```python
from build123d import *

# Parameters (mm, degrees)
F0_R     = 6
F1_DEPTH = 90


with BuildPart() as f1:
    # F0 (on Top) → F1 (new body)
    with BuildSketch(Plane.XY):
        with BuildLine():
            Line((17.5, 125), (17.5, 112.5))
            ThreePointArc((17.5, 112.5), (0, 95), (-17.5, 112.5))
            Line((-17.5, 112.5), (-17.5, 125))
            ThreePointArc((-17.5, 125), (-63.109528, 109.308909), (-99.503175, 77.655445))
            Line((-99.503175, 77.655445), (-88.677858, 71.405445))
            ThreePointArc((-88.677858, 71.405445), (-82.272413, 47.5), (-106.177858, 41.094555))
            Line((-106.177858, 41.094555), (-117.003175, 47.344555))
            ThreePointArc((-117.003175, 47.344555), (-126.219056, 0), (-117.003175, -47.344555))
            Line((-117.003175, -47.344555), (-106.177858, -41.094555))
            ThreePointArc((-106.177858, -41.094555), (-82.272413, -47.5), (-88.677858, -71.405445))
            Line((-88.677858, -71.405445), (-99.503175, -77.655445))
            ThreePointArc((-99.503175, -77.655445), (-63.109528, -109.308909), (-17.5, -125))
            Line((-17.5, -125), (-17.5, -112.5))
            ThreePointArc((-17.5, -112.5), (0, -95), (17.5, -112.5))
            Line((17.5, -112.5), (17.5, -125))
            ThreePointArc((17.5, -125), (63.109528, -109.308909), (99.503175, -77.655445))
            Line((99.503175, -77.655445), (88.677858, -71.405445))
            ThreePointArc((88.677858, -71.405445), (82.272413, -47.5), (106.177858, -41.094555))
            Line((106.177858, -41.094555), (117.003175, -47.344555))
            ThreePointArc((117.003175, -47.344555), (126.219056, 0), (117.003175, 47.344555))
            Line((117.003175, 47.344555), (106.177858, 41.094555))
            ThreePointArc((106.177858, 41.094555), (82.272413, 47.5), (88.677858, 71.405445))
            Line((88.677858, 71.405445), (99.503175, 77.655445))
            ThreePointArc((99.503175, 77.655445), (63.109528, 109.308909), (17.5, 125))
        make_face()
        with Locations((0, -50)):
            Circle(F0_R, mode=Mode.SUBTRACT)
        with Locations((0, 50)):
            Circle(F0_R, mode=Mode.SUBTRACT)
    extrude(amount=F1_DEPTH)


solid = f1.part
```
Geometry: final body of the model. Coordinates: model frame, mm. A direction names the side the tool comes from. Round coordinates to 2 decimals unless told otherwise and drop trailing zeros. Order: outer loops, then holes, each group sorted by start corner. A loop starts at its lowest first (then second) coordinate and runs counter-clockwise, first axis right, second up. Notation, with made-up numbers: (88.25, 19) - (134.25, 19) arc R33 ccw to (134.25, 55) - close; hole circle Ø4 at (69.5, -13). An arc over 180 degrees is marked (long way). Write item = value, one per line. Start each with the question number.
Q1. Pin query (flat end, axial travel): pin 1 (10 mm diameter, centred on y = 120, z = 56.5, fed in from +X); pin 2 (1 mm diameter, centred on y = 54.5, z = 69, fed in from -X); pin 3 (8 mm diameter, centred on x = -63.5, y = 6, fed in from -Z); pin 4 (6.5 mm diameter, centred on y = 116.5, z = 64, fed in from -X). Return the tip coordinate at first contact, or that it passes through.
Q2. Pull-direction query (X, two-part tool) for faces 4 (the flat face through (-111.666, -44.263, 44.37)), 5 (the flat face through (-2, 2, 0)), 6 (the cylindrical face through (-62.52, 109.647, 44.37)); classes: +X half, -X half, draft (parallel to the pull), parting line (faces both ways), or undercut.
Q3. Cut plane A-A on z = 8. Return the cut outline in (x, y).
Q4. Cut plane B-B on x = 0. Return the cut outline in (y, z).
Q5. Access query for faces 1 (the flat face through (94.166, -74.574, 44.37)), 2 (the flat face through (111.666, 44.263, 44.37)), 3 (the flat face through (17.5, -119, 44)). Directions: +Z, -Z, +X, -X, +Y, -Y. A direction counts if a zero-diameter tool reaches every point of the face in a straight line with its end or side. Return the directions, or none.
Q6. Ray query, line 1 (Y direction, x = 0, z = 62); line 2 (X direction, y = -46.5, z = 34.5); line 3 (Y direction, x = -98.5, z = 50). Return the intervals inside material, ascending. Write a range as from..to.
Q7. Cut plane D-D on y = -24. Return the cut outline in (x, z), and give its area (3 significant figures).
Q8. Cut plane C-C on y = 105. Return the cut outline in (x, z), and give its area (3 significant figures).
Outcome:
q1.pin_1 = 52.02
q1.pin_2 = -80.07
q1.pin_3 = 0
q1.pin_4 = -55.73
q2.face_4 = undercut
q2.face_5 = draft
q2.face_6 = -X half
q3.outline = (-117, -47.34) - (-106.18, -41.09) arc R17.5 cw to (-88.68, -71.41) - (-99.5, -77.66) arc R126.22 ccw to (-17.5, -125) - (-17.5, -112.5) arc R17.5 cw to (17.5, -112.5) - (17.5, -125) arc R126.22 ccw to (99.5, -77.66) - (88.68, -71.41) arc R17.5 cw to (106.18, -41.09) - (117, -47.34) arc R126.22 ccw to (117, 47.34) - (106.18, 41.09) arc R17.5 cw to (88.68, 71.41) - (99.5, 77.66) arc R126.22 ccw to (17.5, 125) - (17.5, 112.5) arc R17.5 cw to (-17.5, 112.5) - (-17.5, 125) arc R126.22 ccw to (-99.5, 77.66) - (-88.68, 71.41) arc R17.5 cw to (-106.18, 41.09) - (-117, 47.34) arc R126.22 ccw to start; hole circle Ø12 at (0, -50); hole circle Ø12 at (0, 50)
q4.outline = (-95, 0) - (-56, 0) - (-56, 90) - (-95, 90) - close; (-44, 0) - (44, 0) - (44, 90) - (-44, 90) - close; (56, 0) - (95, 0) - (95, 90) - (56, 90) - close
q5.face_1 = +Z, -Z, +X
q5.face_2 = +Z, -Z, +Y
q5.face_3 = +Z, -Z, -Y
q6.line_1 = -95..-56, -44..44, 56..95
q6.line_2 = -117.34..-115.54, -82.9..-4.87, 4.87..82.9, 115.54..117.34
q6.line_3 = -78.92..-77.08, -38.78..38.78, 77.08..78.92
q7.outline = (-123.92, 0) - (123.92, 0) - (123.92, 90) - (-123.92, 90) - close
q7.area = 22,300 mm^2
q8.outline = (-70.04, 0) - (-15.81, 0) - (-15.81, 90) - (-70.04, 90) - close; (15.81, 0) - (70.04, 0) - (70.04, 90) - (15.81, 90) - close
q8.area = 9,760 mm^2
